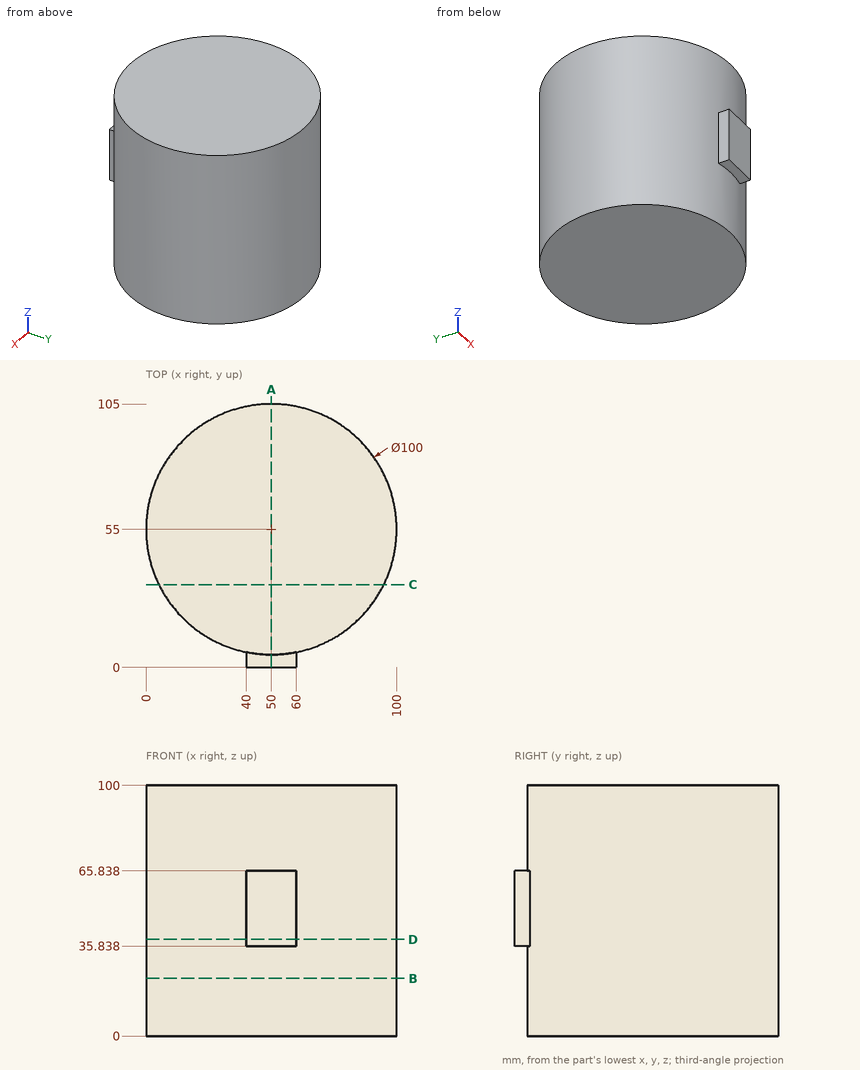
Part print with two shaded views. Sizes in mm from the minimum x, y, z corner. Round coordinates to 2 decimals unless told otherwise and drop trailing zeros. Write each loop counter-clockwise with the first axis right and the second up, starting at its lowest first coordinate (ties: lowest second). Pieces come first, ordered by that corner, then holes. Notation, with made-up numbers: (-3.5, 5) - (43.5, 5) arc R30 ccw to (43.5, 37) - close; hole circle Ø2 at (71, 86.5). An arc over 180 degrees is marked (long way). Use CSV: the item, a comma, the result in double quotes.
Item 1: Slice it at A-A, the plane x = 50. Write the cut outline in (y, z).
Results list:
outline,"(0, 35.84) - (5, 35.84) - (5, 0) - (105, 0) - (105, 100) - (5, 100) - (5, 65.84) - (0, 65.84) - close"
Item 2: Slice it at C-C, the plane y = 33. Write the cut outline in (x, z), then the cut area to 3 significant figures.
Results list:
outline,"(5.1, 0) - (94.9, 0) - (94.9, 100) - (5.1, 100) - close"
area,"8,980 mm²"
Item 3: Wall check: L1, parallel to X at y = 56.5, z = 14; L2, parallel to X at y = 75, z = 8 (1 decimal); L3, parallel to Y at x = 33, z = 81. Give the ranges that are in metal, low to high.
Results list:
L1,"x = 0.02 to 99.98"
L2,"x = 4.2 to 95.8"
L3,"y = 7.98 to 102.02"
Item 4: Flat gauge pins, fed straight in: P1, Ø8, axis at x = 63, y = 17.5, coming from the -Z side; P2, Ø12, axis at y = 63, z = 25, coming from the -X side; P3, Ø5, axis at y = 90, z = 46, coming from the -X side; P4, Ø10, axis at x = 65.5, z = 48, coming from the +Y side (3 decimals). Where does each tip first touch, or does it go through?
Results list:
P1,"stops at z = 0"
P2,"stops at x = 0.04"
P3,"stops at x = 12"
P4,"stops at y = 103.885"
Item 5: Slice it at D-D, the plane z = 38.5. Write the cut outline in (x, y).
Results list:
outline,"(40, 0) - (60, 0) - (60, 6.01) arc R50 ccw (long way) to (40, 6.01) - close"
Item 6: Slice it at B-B, the plane z = 23. Write the cut outline in (x, y).
Results list:
outline,"circle Ø100 at (50, 55)"
